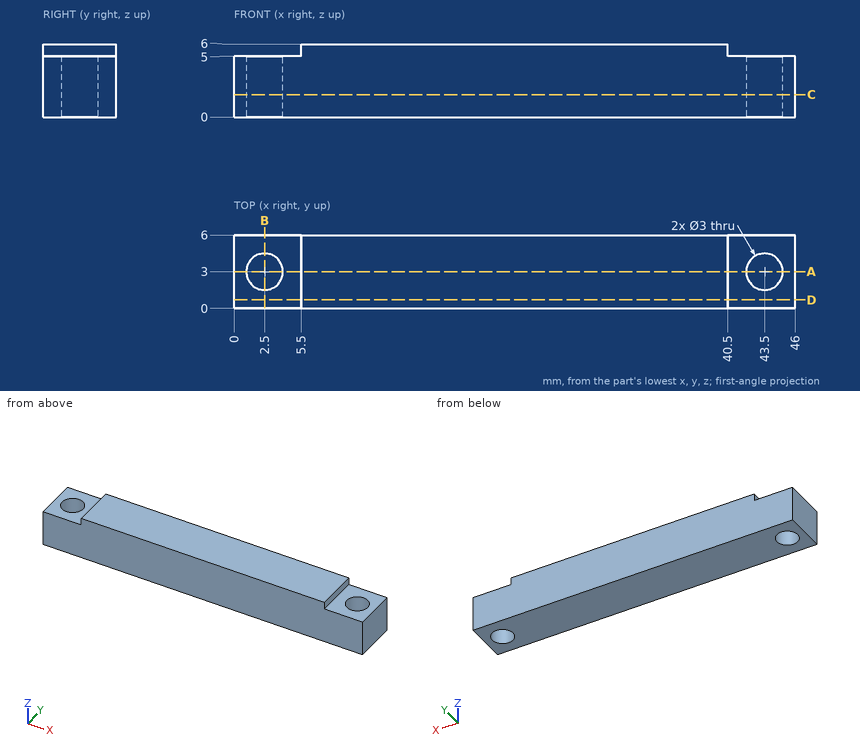
Study the drawing (mm; zero at the part's minimum x, y, z) and answer. Round coordinates to 2 decimals unless told otherwise and drop trailing zeros. Order: outer loops, then holes, each group sorted by start corner. A loop starts at its lowest first (then second) coordinate and runs counter-clockwise, first axis right, second up. Notation, with made-up numbers: M 77,-11.75 L 111,-11.75 A19 cw 111,3.25 Z; hole C 12.25,-9.75 d1. An arc over 180 degrees is marked long. One line per item, written item: value.
Q1. Straight lines are drawn through the part: line 1 (Y direction, x = 43.5, z = 3.5); line 2 (X direction, y = 4.1, z = 2.95); line 3 (Z direction, x = 43, y = 4.45). For each, find the intervals that lie inside material, in ascending order.
Derived:
line 1: 0 to 1.5, 4.5 to 6
line 2: 0 to 1.48, 3.52 to 42.48, 44.52 to 46
line 3: 0 to 5
Q2. Find section C-C on z = 1.85. Write down the section's boundary in (x, y), then the cut area to 3 significant figures.
Derived:
outline: M 0,0 L 46,0 L 46,6 L 0,6 Z; hole C 2.5,3 d3; hole C 43.5,3 d3
area: 262 mm²
Q3. Find section D-D on y = 0.7. Write down the section's boundary in (x, z), then the cut area to 3 significant figures.
Derived:
outline: M 0,0 L 46,0 L 46,5 L 40.5,5 L 40.5,6 L 5.5,6 L 5.5,5 L 0,5 Z
area: 265 mm²
Q4. Find section A-A on y = 3. Write down the section's boundary in (x, z).
Derived:
outline: M 0,0 L 1,0 L 1,5 L 0,5 Z; M 4,0 L 42,0 L 42,5 L 40.5,5 L 40.5,6 L 5.5,6 L 5.5,5 L 4,5 Z; M 45,0 L 46,0 L 46,5 L 45,5 Z
Q5. Find section B-B on x = 2.5. Write down the section's boundary in (y, z).
Derived:
outline: M 0,0 L 1.5,0 L 1.5,5 L 0,5 Z; M 4.5,0 L 6,0 L 6,5 L 4.5,5 Z
